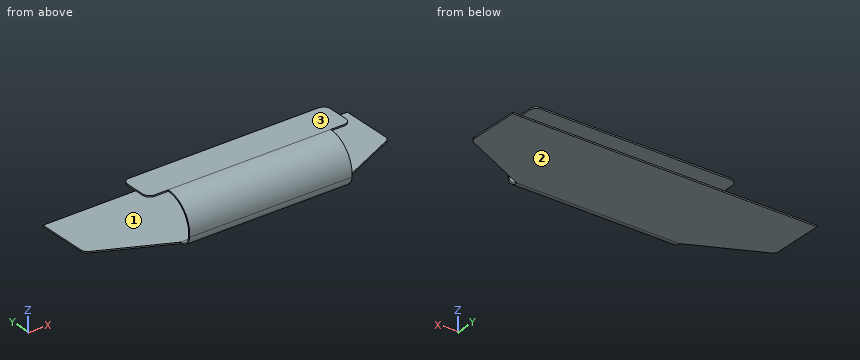
```python
from build123d import *

# Parameters (mm, degrees)
PAD025_DEPTH = 6
PAD026_DEPTH = 0.1
PAD027_DEPTH = 0.1


with BuildPart() as part:
    # Sketch003 → Pad025 (new body, symmetric)
    with BuildSketch(Plane.YZ):
        with BuildLine():
            ThreePointArc((-11.5, 2.9), (-12.972433, 2.255323), (-13.497444, 0.736102))
            ThreePointArc((-13.497444, 0.736102), (-13.242624, 0.212157), (-12.7, 0))
            Line((-12.7, 0), (-12.7, -0.1))
            ThreePointArc((-13.597125, 0.728115), (-13.310452, 0.138677), (-12.7, -0.1))
            ThreePointArc((-11.5, 3), (-13.045913, 2.323151), (-13.597125, 0.728115))
            Line((-11.5, 2.9), (-11.5, 3))
        make_face()
    extrude(amount=PAD025_DEPTH, both=True)

    # Sketch004 → Pad026 (join)
    with BuildSketch(Plane.XY.offset(2.9)):
        with BuildLine():
            Line((-7.5, -9.5), (-7.5, -11))
            ThreePointArc((-7.5, -11), (-7.353553, -11.353553), (-7, -11.5))
            Line((-7, -11.5), (7, -11.5))
            ThreePointArc((7, -11.5), (7.353553, -11.353553), (7.5, -11))
            Line((7.5, -11), (7.5, -9.5))
            ThreePointArc((7.5, -9.5), (7.353553, -9.146447), (7, -9))
            Line((7, -9), (-7, -9))
            ThreePointArc((-7, -9), (-7.353553, -9.146447), (-7.5, -9.5))
        make_face()
    extrude(amount=PAD026_DEPTH)

    # Sketch063 → Pad027 (join)
    with BuildSketch(Plane.XY):
        with BuildLine():
            Line((-6, -12.7), (6, -12.7))
            Line((6, -12.7), (10.963801, -10.351984))
            ThreePointArc((10.963801, -10.351984), (11.172434, -10.167488), (11.25, -9.9))
            Line((11.25, -9.9), (11.25, -6.2))
            Line((11.25, -6.2), (-11.25, -6.2))
            Line((-11.25, -6.2), (-11.25, -9.9))
            ThreePointArc((-11.25, -9.9), (-11.172434, -10.167488), (-10.963801, -10.351984))
            Line((-10.963801, -10.351984), (-6, -12.7))
        make_face()
    extrude(amount=-PAD027_DEPTH)


solid = part.part
```
Geometry: final body of the model. Coordinates: model frame, mm. Face numbers are marked on the shaded views. Coordinates: 2 decimals unless noted, no trailing zeros. Loops run counter-clockwise (first coordinate to the right, second up) from the corner with the lowest first, then second, coordinate; pieces in that order, holes last. Notation, with made-up numbers: (6, -2) -> (10, -2) arc R19 cw to (10, 23) -> close; hole circle Ø1 at (77.5, -19). An arc over 180 degrees is marked (long way). Use a Markdown table: item, result. Add a question column.
(1) Section query C-C, the plane y = -7. Return loops of the section in (x, z).
(2) Section query B-B, the plane y = -10.75. Return loops of the section in (x, z).
(3) Line query: line 1 along Y through (x, z) = (-2, 2.7); line 2 along Y through (x, z) = (3.75, 2.55). Output: solid intervals per line, ascending.
(4) Mould query, pull axis Z, two halves, no side actions, for the marked faces 1, 2 and 3. Classes: pulls with the +Z half, pulls with the -Z half, needs draft (parallel to the pull), parting line crosses it, or undercut.
(5) Section query D-D, the plane z = 1.35. Return loops of the section in (x, y).
(6) Section query A-A, the plane x = 1.5. Return loops of the section in (y, z), plus the area to 3 significant figures.
(7) Pin query (flat end, axial travel): pin 1 Ø1.5 at (x, z) = (-3, 1) entering from +Y. Return the tip coordinate at first contact, or that it passes through.
Answer:
| question | item | result |
|---|---|---|
| 1 | outline | (-11.25, -0.1) -> (11.25, -0.1) -> (11.25, 0) -> (-11.25, 0) -> close |
| 2 | outline | (-10.12, -0.1) -> (10.12, -0.1) -> (10.12, 0) -> (-10.12, 0) -> close; (-7.5, 2.9) -> (7.5, 2.9) -> (7.5, 3) -> (-7.5, 3) -> close |
| 3 | line 1 | y = -12.58 to -12.37 |
| 3 | line 2 | y = -12.8 to -12.63 |
| 4 | face 1 | undercut |
| 4 | face 2 | pulls with the -Z half |
| 4 | face 3 | pulls with the +Z half |
| 5 | outline | (-6, -13.55) -> (6, -13.55) -> (6, -13.45) -> (-6, -13.45) -> close |
| 6 | outline | (-13.6, 0.73) arc R0.9 ccw to (-12.7, -0.1) -> (-6.2, -0.1) -> (-6.2, 0) -> (-12.7, 0) arc R0.8 cw to (-13.5, 0.74) arc R2 cw to (-11.5, 2.9) -> (-9, 2.9) -> (-9, 3) -> (-11.5, 3) arc R2.1 ccw to start |
| 6 | area | 1.37 mm^2 |
| 7 | pin 1 | stops at y = -13.28 |
